Can you work these out from the model? Positions are in its coordinate system, mm. Face numbers are marked on the shaded views. Coordinates: 2 decimals unless noted, no trailing zeros. Order: outer loops, then holes, each group sorted by start corner. A loop starts at its lowest first (then second) coordinate and runs counter-clockwise, first axis right, second up. Notation, with made-up numbers: (-27.75, 55) -> (18.25, 55) arc R12 cw to (18.25, 74) -> close; hole circle Ø5 at (-17.75, -24.5). An arc over 180 degrees is marked (long way). Answer in a Markdown table with one row per item.
```python
from build123d import *

# Parameters (mm, degrees)
CROQUIS1_R              = 6.35
SALIENTE_EXTRUIR1_DEPTH = 30
SALIENTE_EXTRUIR2_DEPTH = 10
CROQUIS4_R              = 6.35
CORTAR_EXTRUIR1_DEPTH   = 43.550949852


with BuildPart() as part:
    # Croquis1 → Saliente-Extruir1 (new body)
    with BuildSketch(Plane.XY):
        Circle(CROQUIS1_R)
    extrude(amount=SALIENTE_EXTRUIR1_DEPTH)

    # Croquis2 → Saliente-Extruir2 (add)
    with BuildSketch(Plane.XY.offset(30)):
        Polygon((10.969655115, 0), (5.484827557, 9.5), (-5.484827557, 9.5), (-10.969655115, 0), (-5.484827557, -9.5), (5.484827557, -9.5), align=None)
    extrude(amount=SALIENTE_EXTRUIR2_DEPTH)

    # Croquis4 → Cortar-Extruir1 (cut, through all)
    with BuildSketch(Plane(origin=(0, 0, 0), x_dir=(-1, 0, 0), z_dir=(0, 0, -1))):
        Circle(CROQUIS4_R)
    extrude(amount=-CORTAR_EXTRUIR1_DEPTH, mode=Mode.SUBTRACT)


solid = part.part
```
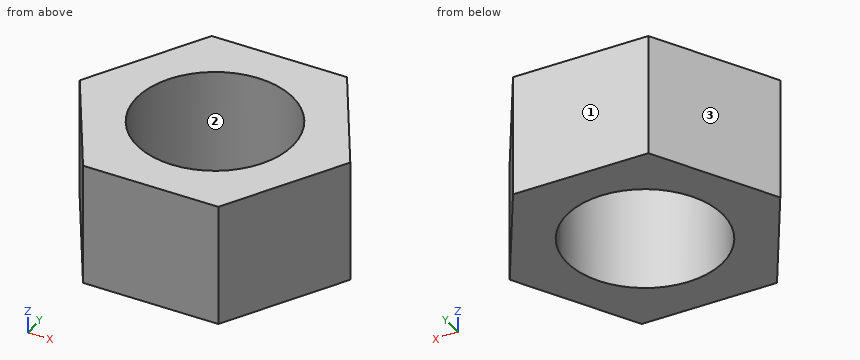
(1) Suppose I cut it at D-D (x = -8.5). Please give me the cut outline in (y, z), and give its area (3 significant figures).
Response values:
| item | result |
|---|---|
| outline | (-4.28, 30) -> (4.28, 30) -> (4.28, 40) -> (-4.28, 40) -> close |
| area | 85.6 mm2 |
(2) I need wall thicknesses on line 1 (Y direction, x = 0, z = 32.5); line 2 (X direction, y = 1.5, z = 35); line 3 (X direction, y = -2, z = 38.25). Which ranges of each line are inside material? Lowest first, please. Write a range as [from, to].
Response values:
| item | result |
|---|---|
| line 1 | [-9.5, -6.35], [6.35, 9.5] |
| line 2 | [-10.1, -6.17], [6.17, 10.1] |
| line 3 | [-9.81, -6.03], [6.03, 9.81] |
(3) Suppose I cut it at A-A (x = 0). Please give me the cut outline in (y, z), and give its area (3 significant figures).
Response values:
| item | result |
|---|---|
| outline | (-9.5, 30) -> (-6.35, 30) -> (-6.35, 40) -> (-9.5, 40) -> close; (6.35, 30) -> (9.5, 30) -> (9.5, 40) -> (6.35, 40) -> close |
| area | 63.0 mm2 |
(4) We'd pull the mould along X, two halves only. Please class the marked faces 1, 2 and 3: +X half, -X half, draft (parallel to the pull), parting line (faces both ways), or undercut.
Response values:
| item | result |
|---|---|
| face 1 | draft |
| face 2 | undercut |
| face 3 | -X half |
(5) Suppose I cut it at B-B (z = 35). Please give me the cut outline in (x, y).
Response values:
| item | result |
|---|---|
| outline | (-10.97, 0) -> (-5.48, -9.5) -> (5.48, -9.5) -> (10.97, 0) -> (5.48, 9.5) -> (-5.48, 9.5) -> close; hole circle Ø12.7 at (0, 0) |
(6) Will these pins go through, and if not, where does the flat tip stop? pin 1 Ø1.5 at (y, z) = (-7.5, 38) entering from +X; pin 2 Ø3 at (y, z) = (1, 34.5) entering from +X.
Response values:
| item | result |
|---|---|
| pin 1 | x = 7.07 |
| pin 2 | x = 10.97 |
(7) Suppose I cut it at C-C (y = -5). Please give me the cut outline in (x, z).
Response values:
| item | result |
|---|---|
| outline | (-8.08, 30) -> (-3.91, 30) -> (-3.91, 40) -> (-8.08, 40) -> close; (3.91, 30) -> (8.08, 30) -> (8.08, 40) -> (3.91, 40) -> close |
